Design review of the part built by this model. Coordinates are the model's own, in mm. A direction names the side the tool comes from. Give positions to 0.01 mm unless a question says otherwise; leave off trailing zeros. Loops run counter-clockwise (first coordinate to the right, second up) from the corner with the lowest first, then second, coordinate; pieces in that order, holes last. Notation, with made-up numbers: M 69.5,79 L 123.5,79 A16 cw 123.5,89 Z; hole C 36,11 d6. An arc over 180 degrees is marked long. Use one line per item in the form item = value. Start each with the question number.
from build123d import *
from build123d.topology import SkipClean

# Parameters (mm, degrees)
BOSS_EXTRUDE1_DEPTH     = 10
SKETCH2_R               = 13.15
SKETCH2_R_2             = 8.15
BOSS_EXTRUDE2_DEPTH     = 13.660254
BOSS_EXTRUDE4_OUTLINE_W = 10
BOSS_EXTRUDE4_OUTLINE_H = 10
BOSS_EXTRUDE4_DEPTH     = 3.254420179


# Read off the part's stored shape, not the designer's step: Boss-Extrude4
with BuildPart() as part:
    # Sketch1 → Boss-Extrude1 (new body)
    with BuildSketch(Plane(origin=(0, 0, 0), x_dir=(1, 0, 0), z_dir=(0, 1, 0))):
        Polygon((-5, -2.85), (-5, 5), (-7.5, 5), (-6.5, 0), (-10, 0), (-10, -2.85), align=None)
        Polygon((0, 0), (-3.5, 0), (-2.5, 5), (-5, 5), (-5, -2.85), (0, -2.85), align=None)
    extrude(amount=BOSS_EXTRUDE1_DEPTH)



with BuildPart() as body_2:
    # Sketch2 → Boss-Extrude2 (new body)
    with BuildSketch(Plane(origin=(4.330127019, 2.5, 0), x_dir=(0, 0, -1), z_dir=(-0.8660254037844362, -0.5000000000000041, 0))):
        with Locations(Location((-16, -8.660254038, 0), (0, 0, 270))):
            Circle(SKETCH2_R)
        with Locations(Location((-16, -8.660254038, 0), (0, 0, 270))):
            Circle(SKETCH2_R_2, mode=Mode.SUBTRACT)
    extrude(amount=BOSS_EXTRUDE2_DEPTH)


with BuildPart() as part_1:
    with SkipClean():  # the faces are left unmerged after this step: merging them gives an invalid solid
        add(part.part)

        add(body_2.part)  # Boss-Extrude4 merges body 2
        # Boss-Extrude4 outline → Boss-Extrude4 (add)
        with BuildSketch(Plane.XY.offset(2.85)):
            with Locations((-5, 5)):
                Rectangle(BOSS_EXTRUDE4_OUTLINE_W, BOSS_EXTRUDE4_OUTLINE_H)
        extrude(amount=BOSS_EXTRUDE4_DEPTH)


solid = part_1.part
Q1. The part is to be moulded in two halves that separate along Y. For faces 4 (the cylindrical face through (-9.719, 13.365, 13.552)), 5 (the flat face through (0, 10, 25)), 6 (the flat face through (-3, 4.9, -2.5)), say which applies: pulls with the +Y half, pulls with the -Y half, needs draft (parallel to the pull), parting line crosses it, or undercut.
Q2. Wall thickness on probe 1 along Z at (x, y) = (-6.25, 6); probe 2 along Z at (x, y) = (-10.75, 2.75); probe 3 along Y at (x, z) = (-5.25, 0): over which ranges is each line inside the solid? List them lowest first.
Q3. Take a section at A-A on z = 15. Give the boundary of the cut face in (x, y).
Q4. Clearance check with flat-ended pins moving along their axes: pin 1 Ø10 at (x, z) = (-9, 7) entering from +Y; pin 2 Ø4 at (x, z) = (-3, -3) entering from -Y; pin 3 Ø3 at (x, y) = (-4.5, -5) entering from -Z. State where each tip first meets the part, or that it passes through.
Q5. Take a section at B-B on z = 22. Give the boundary of the cut face in (x, y), plus the area to 3 significant figures.
Q6. For faces 1 (the flat face through (-7, 4.9, -2.5)), 2 (the flat face through (-11.74, 3.01, 24.58)), 3 (the flat face through (-2, 5, 0)), list the 3-axis set-ups (+Z, -Z, +X, -X, +Y, -Y) from which the entire face can be reached by the end or side of a thin tool; tool diameter is ignored.
Q7. Take a section at C-C on z = 26. Give the boundary of the cut face in (x, y).
Response values:
q1.face_4 = undercut
q1.face_5 = pulls with the +Y half
q1.face_6 = needs draft
q2.probe_1 = -5 to 7.86, 24.14 to 29.15
q2.probe_2 = 2.88 to 7.9, 24.1 to 29.12
q2.probe_3 = 0 to 10
q3.outline = M -18.39,14.53 L -15.87,10.17 L -4.04,17 L -6.56,21.36 Z; M -7.79,-3.83 L -5.27,-8.19 L 6.56,-1.36 L 4.04,3 Z
q4.pin_1 = 20.56
q4.pin_2 = 0
q4.pin_3 = 6.64
q5.outline = M -17.68,13.3 L -14.59,7.95 L -2.76,14.78 L -5.85,20.13 Z; M -9.07,-1.61 L -5.98,-6.96 L 5.85,-0.13 L 2.76,5.22 Z
q5.area = 169 mm^2
q6.face_1 = -X, +Y, -Y
q6.face_2 = +Z, -Z, -X, -Y
q6.face_3 = +X, +Y, -Y
q7.outline = M -16.1,10.57 L -7.56,-4.23 L 4.27,2.6 L -4.27,17.4 Z
